The drawing under review shows one solid part. Ordinate dimensions are in mm from its lowest x, y, z. A direction names the side the tool comes from. Coordinates: 2 decimals unless noted, no trailing zeros. Write each loop counter-clockwise with the first axis right and the second up, starting at its lowest first coordinate (ties: lowest second). Pieces come first, ordered by that corner, then holes. Notation, with made-up numbers: M -30,10 L -16,10 A34 cw -16,42 Z; hole C 8.25,3.25 d11. An arc over 180 degrees is marked long. Write item = value, one per line.
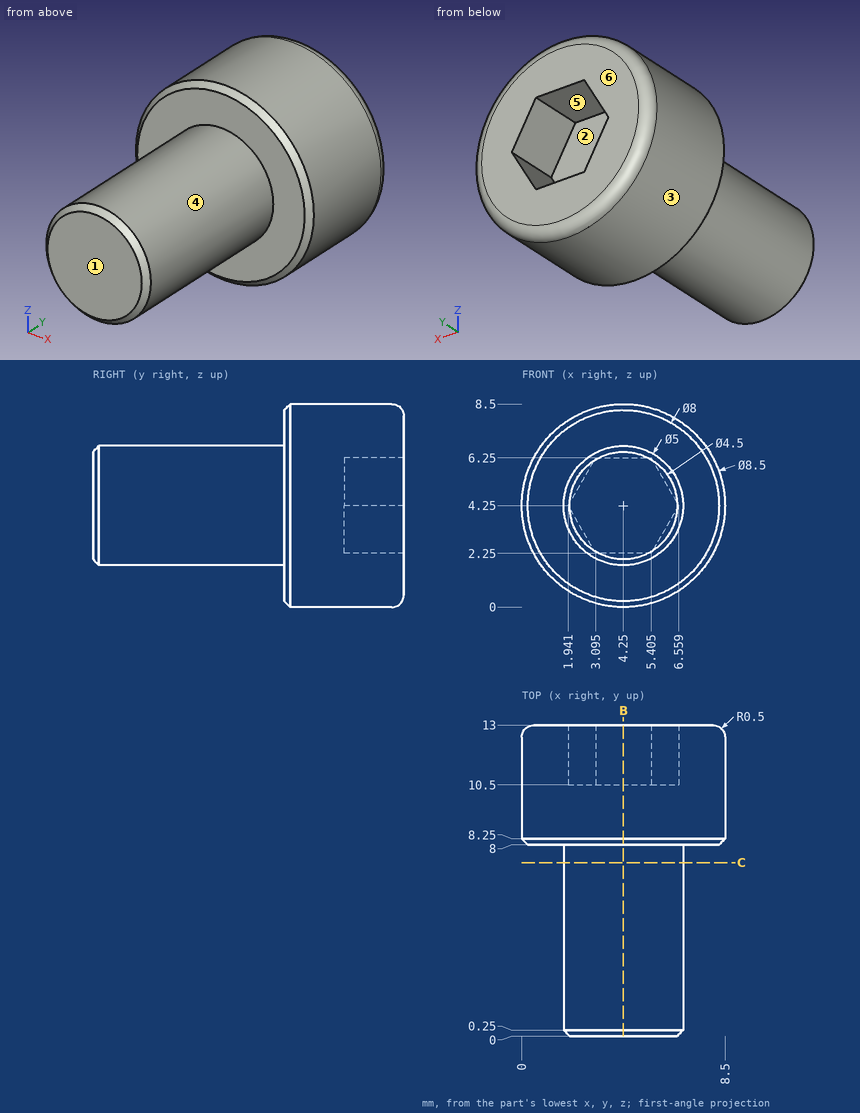
Q1. The part is to be moulded in two halves that separate along X. For the marked faces 1, 2 and 3, say which applies: +X half, -X half, draft (parallel to the pull), parting line (faces both ways), or undercut.
Check result:
face_1 = draft
face_2 = undercut
face_3 = parting line
Q2. For P1, Ø4, axis at x = 3.5, z = 3, coming from the -Y side; P2, Ø1.5, axis at y = 2.5, z = 4, coming from the +X side; P3, Ø1, axis at y = 4.5, z = 4, coming from the -X side; P4, Ø2, axis at x = 5, y = 6.5, coming from the +Z side, all flat-tipped, find the tip position at first contact; note any pin that passes through.
Check result:
P1 = 0
P2 = 6.75
P3 = 1.75
P4 = 6.75
Q3. Wall thickness on line 1 (Y direction, x = 2.5, z = 4.75); line 2 (Z direction, x = 4.25, y = 7.25); line 3 (Y direction, x = 1.75, z = 3): over which ranges is each line inside the solid? List them lowest first.
Check result:
line_1 = 0 to 10.5
line_2 = 1.75 to 6.75
line_3 = 8 to 13
Q4. Consider section B-B, the plane x = 4.25. State the section outline as (y, z) points.
Check result:
outline = M 0,2 L 0.25,1.75 L 8,1.75 L 8,0.25 L 8.25,0 L 12.5,0 A0.5 ccw 13,0.5 L 13,2.25 L 10.5,2.25 L 10.5,6.25 L 13,6.25 L 13,8 A0.5 ccw 12.5,8.5 L 8.25,8.5 L 8,8.25 L 8,6.75 L 0.25,6.75 L 0,6.5 Z
Q5. Machinability: for the marked faces 4, 5 and 6, which of the approach directions +Z, -Z, +X, -X, +Y, -Y give a long, thin tool a straight path to every point of the face, cutting with its end or side? Answer none if there is none.
Check result:
face_4 = -Y
face_5 = +Y
face_6 = +Z, -Z, +X, -X, +Y
Q6. Consider section C-C, the plane y = 7.25. State the section outline as (x, z) points.
Check result:
outline = C 4.25,4.25 d5
